Could you check a few things on this model? Use its own coordinates, in mm. A direction names the side the tool comes from. Coordinates: 2 decimals unless noted, no trailing zeros. Write each loop counter-clockwise with the first axis right and the second up, starting at its lowest first coordinate (ties: lowest second). Pieces come first, ordered by that corner, then holes. Notation, with made-up numbers: M -34.5,-19.75 L -19.5,-19.75 A14 cw -19.5,-0.75 Z; hole C 66,-28 d8. An arc over 180 degrees is marked long. Write item = value, one per line.
```python
from build123d import *

# Parameters (mm, degrees)
SKETCH_1_R               = 3
EXTRUDE_1_DEPTH          = 25
CHAMFER_1_SIZE           = 1
CUT_EXTRUDE_1_DEPTH      = 26.357444666
CUT_EXTRUDE_1_DEPTH_BACK = 26.357444666
CUT_EXTRUDE_2_DEPTH      = 26.357444666
CUT_EXTRUDE_2_DEPTH_BACK = 26.357444666


with BuildPart() as part:
    # 草图1 → 凸台-拉伸1 (new body)
    with BuildSketch(Plane(origin=(0, 0, 0), x_dir=(1, 0, 0), z_dir=(0, 1, 0))):
        with Locations(Location((0, 0, 0), (0, 0, 270))):
            Circle(SKETCH_1_R)
    extrude(amount=EXTRUDE_1_DEPTH)

    # 倒角1
    chamfer_1_edges = [part.edges().sort_by_distance(p)[0] for p in [
        (0, 0, -3),
    ]]
    chamfer(chamfer_1_edges, length=CHAMFER_1_SIZE)

    # 草图2 → 切除-拉伸1 (cut, two sides: drawn at the far end of the back side and taken through both)
    with BuildSketch(Plane.XY.offset(-CUT_EXTRUDE_1_DEPTH_BACK)):
        Polygon((-52.748448143, -11.06198798), (-3, 23.6), (-0.990656871, 25), (48.757791272, 59.66198798), (-20.566184689, 159.158884265), (-122.072424103, 88.434908305), align=None)
    extrude(amount=CUT_EXTRUDE_1_DEPTH + CUT_EXTRUDE_1_DEPTH_BACK, mode=Mode.SUBTRACT)

    # 草图3 → 切除-拉伸2 (cut, two sides: drawn at the far end of the back side and taken through both)
    with BuildSketch(Plane.XY.offset(-CUT_EXTRUDE_2_DEPTH_BACK)):
        Polygon((0, 85.358713248), (0, 25), (0, 21), (3, 21), (63.358713248, 21), (149.384538564, 105.689163643), (86.025825316, 170.047876891), align=None)
    extrude(amount=CUT_EXTRUDE_2_DEPTH + CUT_EXTRUDE_2_DEPTH_BACK, mode=Mode.SUBTRACT)


solid = part.part
```
Item 1: I'm going to push flat-ended pins straight in: P1, Ø2.5, axis at x = 2, z = -1, coming from the +Y side; P2, Ø1.2, axis at y = 23.5, z = 0, coming from the +X side; P3, Ø1, axis at y = 14.5, z = 1, coming from the +X side. Where does each tip first touch, or does it pass through?
Numbers:
P1 = 21
P2 = 0
P3 = 2.96
Item 2: Imagine slicing it at A-A (z = 0). Write out the boundary of the cut face in (x, y).
Numbers:
outline = M -3,1 L -2,0 L 2,0 L 3,1 L 3,21 L 0,21 L 0,25 L -0.99,25 L -3,23.6 Z
Item 3: Imagine slicing it at B-B (y = 18.5). Write out the boundary of the cut face in (x, z).
Numbers:
outline = C 0,0 d6
Item 4: If I drill on line 1 along Y through (x, z) = (0.55, 1.2); line 2 along X through (y, z) = (11.75, -0.1); line 3 along X through (y, z) = (8.75, -1), over which ranges is the centre line in solid material (lowest first)?
Numbers:
line_1 = 0 to 21
line_2 = -3 to 3
line_3 = -2.83 to 2.83
Item 5: For faces 1 (the face through (0, 0, 0)), 2 (the face through (1, 21, 0)), which set-ups out of +Z, -Z, +X, -X, +Y, -Y let a thin tool reach every point of the face, with its end or its side?
Numbers:
face_1 = +Z, -Z, +X, -X, -Y
face_2 = +Z, -Z, +X, +Y
